```python
from build123d import *

# Parameters (mm, degrees)
F1_DEPTH = 25.4
F3_DEPTH = 101.6
F5_DEPTH = 127


with BuildPart() as f1:
    # F0 (on Top) → F1 (new body)
    with BuildSketch(Plane.XY):
        Polygon((32.903377, 31.103013), (-95.314093, 31.103013), (-95.314093, -29.911235), (33.370786, -29.911235), (86.780615, -17.424744), (86.780615, 18.638877), align=None)
    extrude(amount=F1_DEPTH)

    # F2 (on Right) → F3 (join, symmetric)
    with BuildSketch(Plane.YZ):
        Polygon((-13.52687, 44.609893), (-29.9318, 25.902519), (31.083023, 25.326908), (16.404927, 44.322085), align=None)
    extrude(amount=F3_DEPTH, both=True)

    # F4 (on Front) → F5 (cut, symmetric)
    with BuildSketch(Plane.XZ):
        Polygon((33.817593, 0), (86.885192, 0), (110.29736, 0), (110.29736, 60.351387), (87.925732, 60.351387), (13.527044, 60.351387), (86.885192, 25.980785), (86.885192, 12.990392), align=None)
    extrude(amount=F5_DEPTH, both=True, mode=Mode.SUBTRACT)


solid = f1.part
```
CAD build for the part. Positions are in the model's coordinates, mm. A direction names the side the tool comes from. Round coordinates to 2 decimals unless told otherwise and drop trailing zeros. Order: outer loops, then holes, each group sorted by start corner. A loop starts at its lowest first (then second) coordinate and runs counter-clockwise, first axis right, second up.
Item 1: Mould opens along Z. For faces 1 (the face through (-6, -3, 25.4)), 2 (the face through (-6.04, -21.61, 35.39)), 3 (the face through (59.702, -23.755, 15.344)) say: pulls with the +Z half, pulls with the -Z half, needs draft (parallel to the pull), parting line crosses it, or undercut.
Item 2: Saw through at B-B on x = -85. Write the cut outline in (y, z).
Item 3: Pin check, flat tips, straight feed: pin 1 (7.5 mm diameter, centred on y = 4.5, z = 13, fed in from -X); pin 2 (8 mm diameter, centred on x = 8.5, y = -24, fed in from +Z); pin 3 (10 mm diameter, centred on y = -17, z = 26.5, fed in from +X); pin 4 (12 mm diameter, centred on x = 48, y = 3, fed in from +Z). Stop position of each tip, or through.
Item 4: Tool access for faces 4 (the face through (-95.314, 1, 13)), 5 (the face through (60.219, 24.784, 15.344)), 6 (the face through (60.67, 0.117, 6.573)): list every direction of +Z, -Z, +X, -X, +Y, -Y with a clear straight run to the whole face (end or side of a thin tool).
Item 5: Probe line 1 along Y through (x, z) = (-14.5, 21); line 2 along Z through (x, y) = (53, -11.5); line 3 along Z through (x, y) = (-45, -22.5). List the from-to ranges inside material, lowest first.
Item 6: Saw through at A-A on y = -25. Write the cut outline in (x, z).
Item 7: Saw through at C-C on x = 68.5. Write the cut outline in (y, z).
Item 8: Saw through at D-D on z = 20.5. Write the cut outline in (x, y).
Reported:
1. face 1: undercut
1. face 2: pulls with the +Z half
1. face 3: needs draft
2. outline: (-29.93, 25.9) - (23.34, 25.4) - (-29.91, 25.4) - (-29.91, 0) - (31.1, 0) - (31.1, 25.4) - (31.03, 25.4) - (16.4, 44.32) - (-13.53, 44.61) - close
3. pin 1: stops at x = -95.31
3. pin 2: stops at z = 37.23
3. pin 3: stops at x = 86.89
3. pin 4: stops at z = 44.51
4. face 4: -Z, -X, +Y, -Y
4. face 5: -Z, +X, +Y
4. face 6: -Z, +X, +Y, -Y
5. line 1: y = -29.91 to 31.1
5. line 2: z = 4.7 to 25.4, 25.73 to 41.86
5. line 3: z = 0 to 25.4, 25.83 to 34.38
6. outline: (-101.6, 25.86) - (86.89, 25.86) - (86.89, 25.98) - (75.05, 31.53) - (-101.6, 31.53) - close; (-95.31, 0) - (33.82, 0) - (54.38, 5.03) - (54.38, 25.4) - (-95.31, 25.4) - close
7. outline: (-29.93, 25.9) - (31.08, 25.33) - (23.92, 34.59) - (-22.31, 34.59) - close; (-21.7, 8.49) - (22.87, 8.49) - (22.87, 25.4) - (-21.7, 25.4) - close
8. outline: (-95.31, -29.91) - (33.37, -29.91) - (86.78, -17.42) - (86.78, 18.64) - (32.9, 31.1) - (-95.31, 31.1) - close
